```python
from build123d import *

# Parameters (mm, degrees)
SKETCH1_W           = 48
SKETCH1_H           = 28
BOSS_EXTRUDE1_DEPTH = 9
SKETCH2_W           = 45
SKETCH2_H           = 25
CUT_EXTRUDE1_DEPTH  = 8
SKETCH3_R           = 8.5
CUT_EXTRUDE2_DEPTH  = 22
SKETCH4_W           = 46.5
SKETCH4_H           = 26.5
CUT_EXTRUDE3_DEPTH  = 1
SKETCH10_W          = 8
SKETCH10_H          = 3.5
CUT_EXTRUDE4_DEPTH  = 30.206163733
FILLET5_R           = 0.5


with BuildPart() as part:
    # Sketch1 → Boss-Extrude1 (new body)
    with BuildSketch(Plane(origin=(0, 0, 0), x_dir=(1, 0, 0), z_dir=(0, 1, 0))):
        Rectangle(SKETCH1_W, SKETCH1_H)
    extrude(amount=BOSS_EXTRUDE1_DEPTH)

    # Sketch2 → Cut-Extrude1 (cut)
    with BuildSketch(Plane.XZ):
        Rectangle(SKETCH2_W, SKETCH2_H)
    extrude(amount=-CUT_EXTRUDE1_DEPTH, mode=Mode.SUBTRACT)

    # Sketch3 → Cut-Extrude2 (cut)
    with BuildSketch(Plane(origin=(0, 9, 0), x_dir=(1, 0, 0), z_dir=(0, 1, 0))):
        with Locations(Location((-12.95, -2.25, 0), (0, 0, 270))):
            Circle(SKETCH3_R)
        with Locations(Location((12.95, -2.25, 0), (0, 0, 270))):
            Circle(SKETCH3_R)
    extrude(amount=-CUT_EXTRUDE2_DEPTH, mode=Mode.SUBTRACT)

    # Sketch4 → Cut-Extrude3 (cut)
    with BuildSketch(Plane.XZ):
        Rectangle(SKETCH4_W, SKETCH4_H)
    extrude(amount=-CUT_EXTRUDE3_DEPTH, mode=Mode.SUBTRACT)

    # Sketch10 → Cut-Extrude4 (cut, through all)
    with BuildSketch(Plane.XY):
        with Locations((8.5, 1.75)):
            Rectangle(SKETCH10_W, SKETCH10_H)
    extrude(amount=-CUT_EXTRUDE4_DEPTH, mode=Mode.SUBTRACT)

    # Fillet5
    fillet5_edges = [part.edges().sort_by_distance(p)[0] for p in [
        (-24, 9, 0),
        (0, 9, 14),
        (24, 9, 0),
        (0, 9, -14),
        (24, 4.5, 14),
        (-24, 4.5, 14),
        (-24, 4.5, -14),
        (24, 4.5, -14),
    ]]
    fillet(fillet5_edges, radius=FILLET5_R)


solid = part.part
```
Geometry: final body of the model. Coordinates: model frame, mm. A direction names the side the tool comes from. Round coordinates to 2 decimals unless told otherwise and drop trailing zeros. Write each loop counter-clockwise with the first axis right and the second up, starting at its lowest first coordinate (ties: lowest second). Pieces come first, ordered by that corner, then holes. Notation, with made-up numbers: M 35,85.5 L 83,85.5 A26 cw 83,99.5 Z; hole C 58,22 d9. An arc over 180 degrees is marked long. Answer in a Markdown table with one row per item. Add a question column.
(1) Ray query, L1, parallel to X at y = 8.5, z = 2.25; L2, parallel to Z at x = -15, y = 5.75; L3, parallel to X at y = 2.5, z = -10.75. Return the intervals inside material, ascending.
(2) Cut plane B-B, the plane z = -1.75. Return the cut outline in (x, y), then the cut area to 3 significant figures.
(3) Cut plane C-C, the plane x = -12.95. Return the cut outline in (y, z).
(4) Cut plane A-A, the plane y = 6.75. Return the cut outline in (x, z), then the cut area to 3 significant figures.
(5) Contact query for a flat-ended pin moving along its axis: pin 1 (13 mm diameter, centred on x = -7.5, z = -2.5, fed in from -Y). Output: stop coordinate, or through.
(6) Cut plane D-D, the plane y = 2. Return the cut outline in (x, z), then the cut area to 3 significant figures.
(7) Reachability of faces 1 (the face through (17.8, 0.5, -13.25)), 2 (the face through (4.5, 2, -13)), 3 (the face through (0, 4, 14)) from +Z, -Z, +X, -X, +Y, -Y: full face, straight path, thin tool, end or side. Return the list, or none.
Established:
| question | item | result |
|---|---|---|
| 1 | L1 | -24 to -21.45, -4.45 to 4.45, 21.45 to 24 |
| 1 | L2 | -14 to -12.5, 12.5 to 14 |
| 1 | L3 | -24 to -22.5, 22.5 to 24 |
| 2 | outline | M -24,0 L -23.25,0 L -23.25,1 L -22.5,1 L -22.5,8 L -20.45,8 L -20.45,9 L -23.5,9 A0.5 ccw -24,8.5 Z; M -5.45,8 L 5.45,8 L 5.45,9 L -5.45,9 Z; M 20.45,8 L 22.5,8 L 22.5,1 L 23.25,1 L 23.25,0 L 24,0 L 24,8.5 A0.5 ccw 23.5,9 L 20.45,9 Z |
| 2 | area | 40.4 mm² |
| 3 | outline | M 0,-14 L 8.5,-14 A0.5 ccw 9,-13.5 L 9,-6.25 L 8,-6.25 L 8,-12.5 L 1,-12.5 L 1,-13.25 L 0,-13.25 Z; M 0,13.25 L 1,13.25 L 1,12.5 L 8,12.5 L 8,10.75 L 9,10.75 L 9,13.5 A0.5 ccw 8.5,14 L 0,14 Z |
| 4 | outline | M -24,-13.5 A0.5 ccw -23.5,-14 L 23.5,-14 A0.5 ccw 24,-13.5 L 24,13.5 A0.5 ccw 23.5,14 L -23.5,14 A0.5 ccw -24,13.5 Z; hole M -22.5,-12.5 L 22.5,-12.5 L 22.5,12.5 L -22.5,12.5 Z |
| 4 | area | 219 mm² |
| 5 | pin 1 | y = 8 |
| 6 | outline | M -24,-13.5 A0.5 ccw -23.5,-14 L 4.5,-14 L 4.5,-12.5 L -22.5,-12.5 L -22.5,12.5 L 22.5,12.5 L 22.5,-12.5 L 12.5,-12.5 L 12.5,-14 L 23.5,-14 A0.5 ccw 24,-13.5 L 24,13.5 A0.5 ccw 23.5,14 L -23.5,14 A0.5 ccw -24,13.5 Z |
| 6 | area | 207 mm² |
| 7 | face 1 | -Y |
| 7 | face 2 | -Z, -Y |
| 7 | face 3 | +Z, +X, -X, +Y, -Y |
